Check sheet for the modelled part. Datum: model origin and axes. Units: mm. Round coordinates to 2 decimals unless told otherwise and drop trailing zeros. Write each loop counter-clockwise with the first axis right and the second up, starting at its lowest first coordinate (ties: lowest second). Pieces come first, ordered by that corner, then holes.
Item 1: Section check A-A, the plane x = 21.5. Record the cut outline in (y, z).
Item 2: Section check B-B, the plane y = 4.6. Record the cut outline in (x, z).
Item 3: Section check D-D, the plane z = -4.5. Record the cut outline in (x, y).
Item 4: Material ranges on line 1 along Z through (x, y) = (21, 2.3); line 2 along Z through (x, y) = (19.5, 4.1); line 3 along X through (y, z) = (5.1, 28.5), recorded low to high.
Item 5: Depth check by flat-ended pin: pin 1 (1.5 mm diameter, centred on y = 2.5, z = -15, fed in from -X). Enter the tip coordinate at first touch or a pass-through.
Item 6: Section check C-C, the plane x = 17.5. Record the cut outline in (y, z).
Autodesk Inventor part; units mm, degrees
ref_plane "YZ Plane" through (0, 0, 0) normal (1, 0, 0) x (0, 1, 0)
ref_plane "XZ Plane" through (0, 0, 0) normal (0, 1, 0) x (-1, 0, 0)
ref_plane "XY Plane" through (0, 0, 0) normal (0, 0, 1) x (1, 0, 0)
sketch "Sketch1" plane through (0, 0, 0) normal (0, 1, 0) x (-1, 0, 0)
  line L0 (18.6455, 5.0782) -> (18.6456, 5.0782)
  line L1 (-34.5212, -26.5719) -> (-29.8086, -45.0298)
  line L2 (-29.8086, -45.0298) -> (-3.3186, -38.2664)
  circle A0 centre (-21.2762, -8.696) radius 11.176
  line L3 (-8.0312, 50.0415) -> (-8.0312, -19.8085)
  line L4 (-8.0312, -19.8085) -> (-3.3186, -38.2664)
  line L5 (-3.3186, -38.2664) -> (-29.8086, -45.0298)
  line L6 (-29.8086, -45.0298) -> (-34.5212, -26.5719)
  line L7 (-34.5212, -26.5719) -> (-34.5212, 50.0415)
  line L8 (-8.0312, 50.0415) -> (-34.5212, 50.0415)
  point P0 (0, 0)
  dimension "d4" = 22.352
  dimension "d24" = 19.05
  dimension "d25" = 69.85
  dimension "d26" = 19.05
  dimension "d28" = 26.49
  dimension "d29" = 13.245
  dimension "d35" = 58.7375
  dimension "d36" = 75.677
extrude "Extrusion1" add sketch "Sketch1" along normal blind 5.6134
sketch "Sketch2" plane through (0, 5.6134, 0) normal (0, 1, 0) x (1, 0, 0)
  line L0 (34.5212, 26.5719) -> (29.8086, 45.0298)
  line L1 (8.0312, 19.8085) -> (34.5212, 26.5719)
  line L2 (34.5212, 26.5719) -> (33.7735, 29.5006)
  line L3 (33.7735, 29.5006) -> (7.2835, 22.7372)
  line L4 (7.2835, 22.7372) -> (8.0312, 19.8085)
  point P0 (0, 0)
  point P1 (0, 0)
  dimension "d37" = 3.0226
extrude "Extrusion2" cut sketch "Sketch2" against normal blind 3.175
sketch "Sketch3" plane through (0, 5.6134, 0) normal (0, 1, 0) x (1, 0, 0)
  line L0 (33.7735, 29.5006) -> (29.8086, 45.0298)
  line L1 (29.8086, 45.0298) -> (3.3186, 38.2664)
  line L2 (29.8086, 45.0298) -> (34.5212, 26.5719)
  line L3 (29.8086, 45.0298) -> (34.5212, 26.5719)
  line L4 (34.5212, 26.5719) -> (31.8018, 25.8776)
  line L5 (31.8018, 25.8776) -> (27.0891, 44.3355)
  line L6 (27.0891, 44.3355) -> (29.8086, 45.0298)
  point P0 (0, 0)
  point P1 (27.0891, 44.3355)
  dimension "d38" = 2.8067
extrude "Extrusion3" cut sketch "Sketch3" against normal blind 3.175
sketch "Sketch4" plane through (0, 5.6134, 0) normal (0, 1, 0) x (1, 0, 0)
  line L0 (8.0312, -50.0415) -> (34.5212, -50.0415)
  line L1 (34.5212, -50.0415) -> (34.5212, 26.5719)
  circle A0 centre (21.2762, -43.6915) radius 1.6002
  point P0 (0, 0)
  dimension "d30" = 3.2004
  dimension "d31" = 13.245
  dimension "d32" = 6.35
extrude "Extrusion4" cut sketch "Sketch4" against normal blind 25.4
properties part number "Lidar Sensor Case Piece 2"
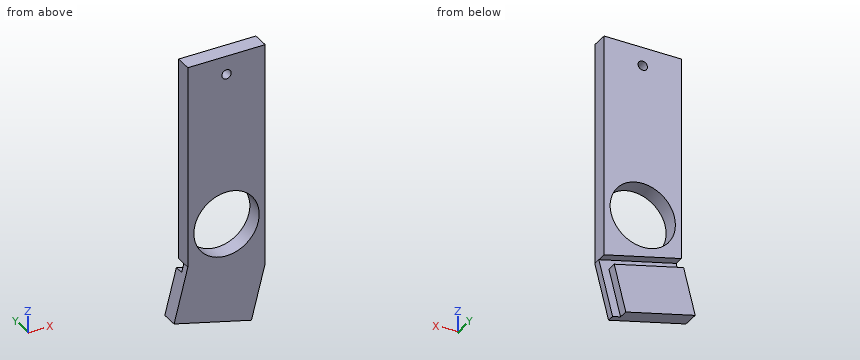
Values found:
1. outline: (0, -42.91) - (5.61, -42.91) - (5.61, -26.37) - (2.44, -26.37) - (2.44, -23.25) - (5.61, -23.25) - (5.61, -19.87) - (0, -19.87) - close; (0, 2.48) - (5.61, 2.48) - (5.61, 42.11) - (0, 42.11) - close; (0, 45.28) - (5.61, 45.28) - (5.61, 50.04) - (0, 50.04) - close
2. outline: (3.32, -38.27) - (27.09, -44.34) - (31.05, -28.81) - (7.28, -22.74) - close; (8.03, -19.81) - (34.52, -26.57) - (34.52, 50.04) - (8.03, 50.04) - close; hole circle Ø22.35 at (21.28, -8.7); hole circle Ø3.2 at (21.28, 43.69)
3. outline: (8.03, 0) - (10.92, 0) - (10.92, 5.61) - (8.03, 5.61) - close; (31.63, 0) - (34.52, 0) - (34.52, 5.61) - (31.63, 5.61) - close
4. line 1: z = -42.78 to -19.87, 2.48 to 42.12, 45.27 to 50.04
4. line 2: z = -42.4 to -25.86, -22.74 to -19.73, 2.34 to 50.04
4. line 3: x = 8.03 to 34.52
5. pin 1: stops at x = 8.03
6. outline: (0, -41.89) - (5.61, -41.89) - (5.61, -25.35) - (2.44, -25.35) - (2.44, -22.23) - (5.61, -22.23) - (5.61, -19.21) - (0, -19.21) - close; (0, 1.82) - (5.61, 1.82) - (5.61, 50.04) - (0, 50.04) - close
